Autodesk Inventor part; units mm, degrees
ref_plane "YZ Plane" through (0, 0, 0) normal (1, 0, 0) x (0, 1, 0)
ref_plane "XZ Plane" through (0, 0, 0) normal (0, 1, 0) x (-1, 0, 0)
ref_plane "XY Plane" through (0, 0, 0) normal (0, 0, 1) x (1, 0, 0)
sketch "Sketch1" plane through (0, 0, 0) normal (1, 0, 0) x (0, 1, 0)
  line L0 (0, 0) -> (-100, 0)
  line L1 (-100, 0) -> (-100, -150)
  line L2 (-100, -150) -> (0, -150)
  line L3 (0, -150) -> (0, 0)
  dimension "d0" = 100
  dimension "d1" = 150
extrude "Extrusion1" add sketch "Sketch1" along normal blind 15
sketch "Sketch2" plane through (0, -100, 0) normal (0, 0, 1) x (1, 0, 0)
  line L0 (0, 100) -> (0, 0)
  line L1 (0, 100) -> (0, 0)
  line L2 (0, 0) -> (0, 19)
  line L3 (0, 100) -> (0, 81)
  line L4 (0, 81) -> (0, 75)
  line L5 (0, 75) -> (0, 69)
  circle A0 centre (0, 75) radius 6
  line L6 (0, 69) -> (0, 56)
  line L7 (0, 56) -> (0, 50)
  circle A1 centre (0, 50) radius 6
  line L8 (0, 44) -> (0, 31)
  line L9 (0, 31) -> (0, 25)
  circle A2 centre (0, 25) radius 6
  dimension "d11" = 12
  dimension "d4" = 19
  dimension "d5" = 19
  dimension "d6" = 6
  dimension "d7" = 6
  dimension "d8" = 12
  dimension "d9" = 13
  dimension "d10" = 6
  dimension "d12" = 13
  dimension "d13" = 6
  dimension "d14" = 12
extrude "Extrusion2" add sketch "Sketch2" along normal blind 680
sketch "Sketch3" plane through (0, -25, 680) normal (0, 0, 1) x (1, 0, 0)
  line L0 (0, -75) -> (0, 25)
  line L1 (15, 25) -> (15, -75)
  line L2 (0, 25) -> (15, 25)
  line L3 (15, 25) -> (15, -75)
  line L4 (15, -75) -> (0, -75)
  line L5 (0, -75) -> (0, 25)
extrude "Extrusion3" add sketch "Sketch3" along normal blind 150
sketch "Sketch4" plane through (15, -100, 680) normal (1, 0, 0) x (0, 0, -1)
  line L0 (0, 100) -> (-150, 100)
  line L1 (830, 0) -> (830, 100)
  line L2 (-150, 100) -> (830, 100)
  line L3 (830, 100) -> (830, 0)
  line L4 (830, 0) -> (-150, 0)
  line L5 (-150, 0) -> (-150, 100)
  point P0 (680, 100)
extrude "Extrusion4" add sketch "Sketch4" along normal blind 100
sketch "Sketch5" plane through (0, 0, 0) normal (0, 1, 0) x (1, 0, 0)
  line L0 (15, -680) -> (0, -680)
  line L1 (15, -680) -> (58.7284, -680)
  line L2 (58.7284, -680) -> (58.7284, 0)
  line L3 (58.7284, 0) -> (15, 0)
  line L4 (15, 0) -> (15, -680)
  point P0 (0, 0)
extrude "Extrusion5" cut sketch "Sketch5" along normal through all both and the other way through all
properties part number "support"
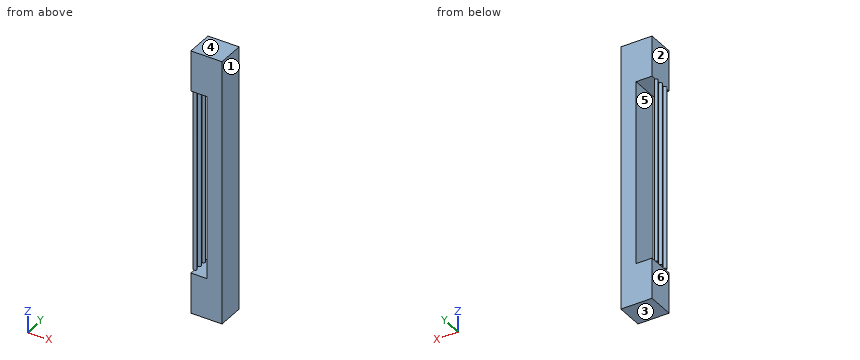
Part model, mm, in its own coordinate system. Face numbers are marked on the shaded views. A direction names the side the tool comes from. Coordinates: 2 decimals unless noted, no trailing zeros. Loops run counter-clockwise (first coordinate to the right, second up) from the corner with the lowest first, then second, coordinate; pieces in that order, holes last. Notation, with made-up numbers: M 85.5,6.5 L 96.5,6.5 A27 ccw 96.5,30.5 Z; hole C 57.5,48 d7. An arc over 180 degrees is marked long. Use a Markdown table: item, result. Add a question column.
Q1. Cut at A-A (z = 348). Write the cut outline in (x, y).
Q2. Pin check, flat tips, straight feed: P1, Ø6.5, axis at x = -2, y = -27.5, coming from the -Z side; P2, Ø10, axis at x = 10, z = 447, coming from the -Y side; P3, Ø6.5, axis at x = -3.5, y = -49.5, coming from the +Z side; P4, Ø1.8, axis at x = -4.5, y = -49, coming from the -Z side. Stop position of each tip, or through.
Q3. Cut at B-B (x = 20). Write the cut outline in (y, z).
Q4. Which spindle directions (+Z, -Z, +X, -X, +Y, -Y) get a long thin tool onto all of the face, cutting with end or side? Do the marked faces 1 and 2. Say none if no direction does.
Q5. Mould opens along Z. For the marked faces 3, 4, 5 and 6 say: +Z half, -Z half, draft (parallel to the pull), parting line (faces both ways), or undercut.
Q6. Probe L1, parallel to Z at x = 5, y = -14.5; L2, parallel to Y at x = 2, z = 531.5; L3, parallel to Y at x = 2.5, z = 400.5. List the from-to ranges inside material, lowest first.
Worked out:
| question | item | result |
|---|---|---|
| 1 | outline | C 0,-75 d12; C 0,-50 d12; C 0,-25 d12; M 58.73,-100 L 115,-100 L 115,0 L 58.73,0 Z |
| 2 | P1 | stops at z = -150 |
| 2 | P2 | stops at y = -78.32 |
| 2 | P3 | stops at z = 680 |
| 2 | P4 | stops at z = 0 |
| 3 | outline | M -100,-150 L 0,-150 L 0,0 L -100,0 Z; M -100,680 L 0,680 L 0,830 L -100,830 Z |
| 4 | face 1 | +Z, -Z, +X, +Y, -Y |
| 4 | face 2 | +Z, -X, +Y, -Y |
| 5 | face 3 | -Z half |
| 5 | face 4 | +Z half |
| 5 | face 5 | undercut |
| 5 | face 6 | draft |
| 6 | L1 | z = -150 to 0, 680 to 830 |
| 6 | L2 | y = -80.66 to -69.34, -55.66 to -44.34, -30.66 to -19.34 |
| 6 | L3 | y = -80.45 to -69.55, -55.45 to -44.55, -30.45 to -19.55 |
